For this review, take the finished solid that the model builds, in its own axes (mm). A direction names the side the tool comes from. Give positions to 0.01 mm unless a question says otherwise; leave off trailing zeros. Order: outer loops, then holes, each group sorted by start corner. A loop starts at its lowest first (then second) coordinate and runs counter-clockwise, first axis right, second up. Notation, with made-up numbers: (3, 44.25) - (27, 44.25) arc R24 ccw to (27, 81.25) - close; hole circle Ø10 at (35, 48). An arc over 180 degrees is marked (long way). Use a Markdown table: item, result. Add a question column.
1) Wall thickness on L1, parallel to Z at x = -2, y = 4; L2, parallel to Z at x = -20, y = 5.25; L3, parallel to Z at x = 54, y = 2.5: over which ranges is each line inside the solid? List them lowest first.
2) Clearance check with flat-ended pins moving along their axes: P1, Ø2, axis at y = 4.5, z = -5, coming from the +X side; P2, Ø4.5, axis at x = -21.48, z = -21.5, coming from the -Y side; P3, Ø1.9, axis at y = 1.5, z = -30, coming from the -X side; P4, Ø0.7, axis at y = 5.5, z = -15.5, coming from the -X side. State where each tip first meets the part, or that it passes through.
3) Mouldability with a two-part tool opening along X and no side actions: class faces 1 (the face through (28, 5, -25.796)), 2 (the face through (123.01, 1.22, -34.72)), 3 (the face through (11, 2.4, -22)), 4 (the face through (-40.166, 1.217, -34.718)) as released by +X, released by -X, zero draft, split by the parting line, or undercut.
4) We need section A-A on y = 6. Write out the cut boundary in (x, z), then the cut area to 3 significant figures.
5) We need section B-B on x = 45. Write out the cut boundary in (y, z), then the cut area to 3 significant figures.
6) Machinability: for faces 5 (the face through (40, 5, -36.596)), 6 (the face through (92, 1, -32.146)), 7 (the face through (118, 2.4, -22)), which of the approach directions +Z, -Z, +X, -X, +Y, -Y give a long, thin tool a straight path to every point of the face, cutting with its end or side? Answer none if there is none.
```python
from build123d import *

# Parameters (mm, degrees)
SKETCH1_W               = 172.2
SKETCH1_H               = 35
BOSS_EXTRUDE1_DEPTH     = 2.4
SKETCH2_R               = 1.13
SKETCH2_R_2             = 3.625
SKETCH2_R_3             = 0.5
SKETCH2_W               = 40
SKETCH2_H               = 20
CUT_EXTRUDE1_DEPTH      = 2.4
SKETCH4_W               = 4
SKETCH4_H               = 6
CUT_EXTRUDE2_DEPTH      = 2.4
SKETCH5_W               = 0.5
SKETCH5_H               = 7.5
BOSS_EXTRUDE2_DEPTH     = 0.5
CUT_EXTRUDE3_DEPTH      = 134.373649476
CUT_EXTRUDE3_DEPTH_BACK = 134.373649476
SKETCH7_W               = 41.3
SKETCH7_H               = 21.3
SKETCH7_W_2             = 40
SKETCH7_H_2             = 20
SKETCH8_W               = 124
SKETCH8_H               = 2.4
SKETCH8_W_2             = 64
BOSS_EXTRUDE3_DEPTH     = 5
FILLET1_R               = 15
FILLET2_R               = 2
FILLET3_R               = 1


with BuildPart() as part:
    # Sketch1 → Boss-Extrude1 (new body)
    with BuildSketch(Plane(origin=(0, 0, 0), x_dir=(1, 0, 0), z_dir=(0, 1, 0))):
        with Locations((41.422946176, 21.495750708)):
            Rectangle(SKETCH1_W, SKETCH1_H)
    extrude(amount=BOSS_EXTRUDE1_DEPTH)

    # Sketch2 → Cut-Extrude1 (cut)
    with BuildSketch(Plane(origin=(0, 2.4, 0), x_dir=(1, 0, 0), z_dir=(0, 1, 0))):
        with Locations(Location((67.522946176, 26.495750708, 0), (0, 0, 270))):
            Circle(SKETCH2_R)
        with Locations(Location((117.522946176, 26.495750708, 0), (0, 0, 270))):
            Circle(SKETCH2_R)
        with Locations(Location((117.522946176, 16.495750708, 0), (0, 0, 90))):
            Circle(SKETCH2_R)
        with Locations(Location((67.522946176, 16.495750708, 0), (0, 0, 90))):
            Circle(SKETCH2_R)
        with Locations(Location((-21.477053824, 21.495750708, 0), (0, 0, 270))):
            Circle(SKETCH2_R_2)
        with Locations(Location((-28.907053824, 21.495750708, 0), (0, 0, 270))):
            Circle(SKETCH2_R_3)
        with Locations(Location((-31.842053824, 21.495750708, 0), (0, 0, 270))):
            Circle(SKETCH2_R_3)
        with Locations(Location((-34.847053824, 21.495750708, 0), (0, 0, 270))):
            Circle(SKETCH2_R_3)
        with Locations(Location((-25.192053824, 27.930319458, 0), (0, 0, 270))):
            Circle(SKETCH2_R_3)
        with Locations(Location((-28.162053824, 33.074510357, 0), (0, 0, 270))):
            Circle(SKETCH2_R_3)
        with Locations(Location((-26.659553824, 30.472104018, 0), (0, 0, 270))):
            Circle(SKETCH2_R_3)
        with Locations(Location((-17.762053824, 27.930319458, 0), (0, 0, 270))):
            Circle(SKETCH2_R_3)
        with Locations(Location((-14.792053824, 33.074510357, 0), (0, 0, 270))):
            Circle(SKETCH2_R_3)
        with Locations(Location((-16.294553824, 30.472104018, 0), (0, 0, 270))):
            Circle(SKETCH2_R_3)
        with Locations(Location((-14.047053824, 21.495750708, 0), (0, 0, 270))):
            Circle(SKETCH2_R_3)
        with Locations(Location((-8.107053824, 21.495750708, 0), (0, 0, 270))):
            Circle(SKETCH2_R_3)
        with Locations(Location((-11.112053824, 21.495750708, 0), (0, 0, 270))):
            Circle(SKETCH2_R_3)
        with Locations(Location((-17.762053824, 15.061181958, 0), (0, 0, 270))):
            Circle(SKETCH2_R_3)
        with Locations(Location((-14.792053824, 9.91699106, 0), (0, 0, 270))):
            Circle(SKETCH2_R_3)
        with Locations(Location((-16.294553824, 12.519397398, 0), (0, 0, 270))):
            Circle(SKETCH2_R_3)
        with Locations(Location((-25.192053824, 15.061181958, 0), (0, 0, 270))):
            Circle(SKETCH2_R_3)
        with Locations(Location((-28.162053824, 9.91699106, 0), (0, 0, 270))):
            Circle(SKETCH2_R_3)
        with Locations(Location((-26.659553824, 12.519397398, 0), (0, 0, 270))):
            Circle(SKETCH2_R_3)
        with Locations((92.522946176, 21.495750708)):
            Rectangle(SKETCH2_W, SKETCH2_H)
    extrude(amount=-CUT_EXTRUDE1_DEPTH, mode=Mode.SUBTRACT)

    # Sketch4 → Cut-Extrude2 (cut)
    with BuildSketch(Plane(origin=(0, 2.4, 0), x_dir=(1, 0, 0), z_dir=(0, 1, 0))):
        with Locations((114.522946176, 21.495750708)):
            Rectangle(SKETCH4_W, SKETCH4_H)
    extrude(amount=-CUT_EXTRUDE2_DEPTH, mode=Mode.SUBTRACT)

    # Sketch5 → Boss-Extrude2 (add)
    with BuildSketch(Plane(origin=(0, 2.4, 0), x_dir=(1, 0, 0), z_dir=(0, 1, 0))):
        with Locations((102.522946176, 35.245750708)):
            Rectangle(SKETCH5_W, SKETCH5_H)
        with Locations((102.522946176, 7.745750708)):
            Rectangle(SKETCH5_W, SKETCH5_H)
        with Locations((-21.477053824, 7.745750708)):
            Rectangle(SKETCH5_W, SKETCH5_H)
        with Locations((-21.477053824, 35.245750708)):
            Rectangle(SKETCH5_W, SKETCH5_H)
    extrude(amount=BOSS_EXTRUDE2_DEPTH)

    # Sketch7 → Cut-Extrude3 (cut, two sides: drawn at the far end of the back side and taken through both)
    with BuildSketch(Plane(origin=(0, 2.4, 0), x_dir=(1, 0, 0), z_dir=(0, 1, 0)).offset(-CUT_EXTRUDE3_DEPTH_BACK)):
        with Locations((92.522946176, 21.495750708)):
            Rectangle(SKETCH7_W, SKETCH7_H)
        with Locations((92.522946176, 21.495750708)):
            Rectangle(SKETCH7_W_2, SKETCH7_H_2, mode=Mode.SUBTRACT)
    extrude(amount=CUT_EXTRUDE3_DEPTH + CUT_EXTRUDE3_DEPTH_BACK, mode=Mode.SUBTRACT)

    # Sketch8 → Boss-Extrude3 (add)
    with BuildSketch(Plane(origin=(0, 2.4, 0), x_dir=(1, 0, 0), z_dir=(0, 1, 0))):
        with Locations((40.522946176, 37.795750708)):
            Rectangle(SKETCH8_W, SKETCH8_H)
        with Locations((28.743410163, 26.995750708)):
            Rectangle(SKETCH8_W_2, SKETCH8_H)
        with Locations((28.743410163, 15.995750708)):
            Rectangle(SKETCH8_W_2, SKETCH8_H)
        with Locations((40.522946176, 5.195750708)):
            Rectangle(SKETCH8_W, SKETCH8_H)
    extrude(amount=BOSS_EXTRUDE3_DEPTH)

    # Fillet1
    fillet1_edges = [part.edges().sort_by_distance(p)[0] for p in [
        (-44.677053824, 1.2, -38.995750708),
        (127.522946176, 1.2, -38.995750708),
        (127.522946176, 1.2, -3.995750708),
        (-44.677053824, 1.2, -3.995750708),
    ]]
    fillet(fillet1_edges, radius=FILLET1_R)

    # Fillet2
    fillet2_edges = [part.edges().sort_by_distance(p)[0] for p in [
        (113.172946176, 1.2, -18.495750708),
        (113.172946176, 1.2, -24.495750708),
    ]]
    fillet(fillet2_edges, radius=FILLET2_R)

    # Fillet3
    fillet3_edges = [part.edges().sort_by_distance(p)[0] for p in [
        (40.522946176, 2.4, -6.395750708),
        (60.743410163, 2.4, -15.995750708),
        (28.743410163, 2.4, -17.195750708),
        (60.743410163, 2.4, -26.995750708),
        (28.743410163, 2.4, -28.195750708),
        (28.743410163, 2.4, -14.795750708),
        (-3.256589837, 2.4, -15.995750708),
        (-3.256589837, 2.4, -26.995750708),
        (28.743410163, 2.4, -25.795750708),
        (40.522946176, 2.4, -36.595750708),
    ]]
    fillet(fillet3_edges, radius=FILLET3_R)


solid = part.part
```
Checked values:
| question | item | result |
|---|---|---|
| 1 | L1 | -39 to -36.6, -28.2 to -25.8, -17.2 to -14.8, -6.4 to -4 |
| 1 | L2 | -39 to -36.6, -6.4 to -4 |
| 1 | L3 | -39 to -36.03, -28.76 to -25.23, -17.76 to -14.23, -6.96 to -4 |
| 2 | P1 | x = 102.52 |
| 2 | P2 | through |
| 2 | P3 | x = -43.8 |
| 2 | P4 | x = -3.26 |
| 3 | face 1 | zero draft |
| 3 | face 2 | released by +X |
| 3 | face 3 | undercut |
| 3 | face 4 | released by -X |
| 4 | outline | (-21.48, -39) - (102.52, -39) - (102.52, -36.6) - (-21.48, -36.6) - close; (-21.48, -6.4) - (102.52, -6.4) - (102.52, -4) - (-21.48, -4) - close; (-3.26, -28.2) - (60.74, -28.2) - (60.74, -25.8) - (-3.26, -25.8) - close; (-3.26, -17.2) - (60.74, -17.2) - (60.74, -14.8) - (-3.26, -14.8) - close |
| 4 | area | 902 mm² |
| 5 | outline | (0, -39) - (7.4, -39) - (7.4, -36.6) - (3.4, -36.6) arc R1 cw to (2.4, -35.6) - (2.4, -29.2) arc R1 cw to (3.4, -28.2) - (7.4, -28.2) - (7.4, -25.8) - (3.4, -25.8) arc R1 cw to (2.4, -24.8) - (2.4, -18.2) arc R1 cw to (3.4, -17.2) - (7.4, -17.2) - (7.4, -14.8) - (3.4, -14.8) arc R1 cw to (2.4, -13.8) - (2.4, -7.4) arc R1 cw to (3.4, -6.4) - (7.4, -6.4) - (7.4, -4) - (0, -4) - close |
| 5 | area | 133 mm² |
| 6 | face 5 | +X, -X, +Y |
| 6 | face 6 | +Y, -Y |
| 6 | face 7 | +Z, -Z, +X, +Y |
